Can you work these out from the drawing? Everything is in mm from the part's minimum corner. Coordinates: 2 decimals unless noted, no trailing zeros. Loops run counter-clockwise (first coordinate to the right, second up) from the corner with the lowest first, then second, coordinate; pieces in that order, holes last. Notation, with made-up numbers: (-13, -5.5) - (28, -5.5) arc R21 ccw to (28, 10.5) - close; hole circle Ø10 at (-35, -32.5). An arc over 180 degrees is marked (long way). One line per question, with ' | ' between items. Start each with the question number.
1. I want a section at A-A, the plane z = 87. Count the separate pieces of the cut face and the enclosed holes in it, then the cut area to 3 significant figures.
2. Please list where these lines run through material, in increasing order: L1, parallel to Z at x = 12, y = 1.75; L2, parallel to Z at x = 8, y = 3.75 (1 decimal); L3, parallel to X at y = 2.5, z = 96.5 (1 decimal). Write a range as [from, to].
3. I want a section at C-C, the plane z = 12. Write out the boundary of the cut face in (x, y).
4. I'm going to push a flat-ended pin straight in: P1, Ø8.5, axis at x = 11.11, z = 88.9, coming from the +Y side. Where does the tip first touch, or does it pass through?
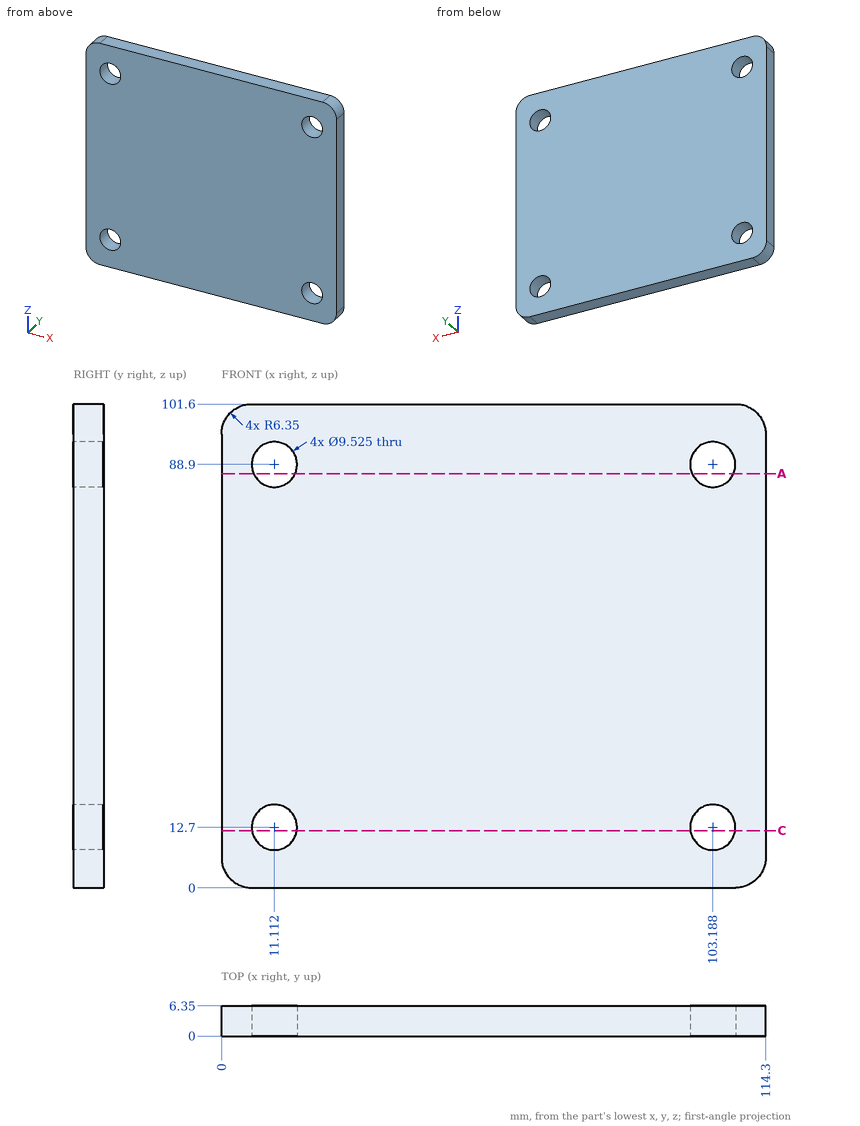
Results are:
1) separate pieces: 3 | enclosed holes: 0 | area: 615 mm2
2) L1: z = [0, 8.02], [17.38, 84.22], [93.58, 101.6] | L2: z = [0, 9.1], [16.3, 85.3], [92.5, 101.6] | L3: x = [0.1, 114.2]
3) outline: (0, 0) - (6.4, 0) - (6.4, 6.35) - (0, 6.35) - close; (15.82, 0) - (98.48, 0) - (98.48, 6.35) - (15.82, 6.35) - close; (107.9, 0) - (114.3, 0) - (114.3, 6.35) - (107.9, 6.35) - close
4) P1: passes through
